Read the model definition and answer for the solid it produces. Units are mm, in the model's axes. A direction names the side the tool comes from. Give positions to 0.01 mm unless a question says otherwise; leave off trailing zeros. Write each loop counter-clockwise with the first axis right and the second up, starting at its lowest first coordinate (ties: lowest second). Pieces come first, ordered by that corner, then holes. Notation, with made-up numbers: (82, 61) -> (111, 61) arc R23 ccw to (111, 71) -> close; hole circle Ø11 at (14.25, 80.5). An arc over 180 degrees is marked (long way). Answer as CSV lines item,"result". Start each with the question number.
1. The part is cut by section B-B, the plane z = -36.5. Determine the outline of the cut face in (x, y), and give its area (3 significant figures).
2. Find the intervals of material crossed by line 1 (Z direction, x = 14.5, y = -16.5); line 2 (Y direction, x = -3.5, z = 11); line 3 (Y direction, x = -6.5, z = 0), in increasing order.
3. A tool of negligible diameter and unlimited length cuts with its end or side. For faces 1 (the flat face through (17, 0, 27)), 2 (the cylindrical face through (-19.535, 0.325, 29.423)), 3 (the cylindrical face through (0.325, 19.535, 29.423)), 4 (the flat face through (-7, -18, 32.845)), 5 (the cylindrical face through (-0.325, -19.535, 29.423)), from which of +Z, -Z, +X, -X, +Y, -Y can it reach the whole face along a straight path? Write none if from no direction.
4. Given pin 1 (6.5 mm diameter, centred on y = 0, z = 26.94, fed in from +X); pin 2 (2.5 mm diameter, centred on y = -1, z = 27, fed in from +X); pin 3 (4.5 mm diameter, centred on x = 0, z = 26.94, fed in from -Y); pin 4 (6 mm diameter, centred on x = -1, y = -1.5, fed in from +Z), each flat-ended and moving along its own axis, determine where each tip first touches the part or whether it passes through.
5. For a pull along X with two mould halves and no side action, classify faces 6 (the conical face through (10.92, -3.44, 23.22)), 7 (the cylindrical face through (19.535, -0.325, 29.423)), 8 (the cylindrical face through (20.32, 8.43, 26.24)) as pulls with the +X half, pulls with the -X half, needs draft (parallel to the pull), parting line crosses it, or undercut.
6. The part is cut by section A-A, the plane z = -15. Determine the outline of the cut face in (x, y).
from build123d import *

# Parameters (mm, degrees)
FILETE5_R             = 1
ESBO_O2_R             = 2.5
CORTE_EXTRUS_O1_DEPTH = 5
PADR_OCIRCULAR1_COUNT = 4
FILETE6_R             = 5
FILETE7_R             = 1
FILETE8_R             = 2


with BuildPart() as part:
    # Esbo_o1 → Revolu_o1 (revolve)
    with BuildSketch(Plane(origin=(0, 0, 0), x_dir=(1, 0, 0), z_dir=(0, 1, 0)), mode=Mode.PRIVATE) as revolu_o1_sk:
        Polygon((-7, -12.473975434), (-15, 48.292057468), (-18.025886882, 48.292057468), (-10.025886882, -12.473975434), (-22, -19.444538182), (-22, -32.844538182), (-19, -32.844538182), (-19, -36.444538182), (-22, -36.444538182), (-22, -41.444538182), (-19, -41.444538182), align=None)
    revolve(revolu_o1_sk.sketch.rotate(Axis((0, 0, 0), (0, 0, -1)), 180), axis=Axis((0, 0, 0), (0, 0, -1)))

    # Filete5
    filete5_edges = [part.edges().sort_by_distance(p)[0] for p in [
        (-7, 0, 12.473975434),
    ]]
    fillet(filete5_edges, radius=FILETE5_R)

    # Esbo_o2 → Corte-extrus_o1 (cut)
    with BuildSketch(Plane.ZX.offset(22)):
        with Locations(Location((26.944538182, 0, 0), (0, 0, 270))):
            Circle(ESBO_O2_R)
    corte_extrus_o1 = extrude(amount=-CORTE_EXTRUS_O1_DEPTH, mode=Mode.SUBTRACT)

    # Padr_oCircular1: Corte-extrus_o1 ×4 about axis
    padr_ocircular1_axis = Axis((0, 0, 0), (0, 0, 1))
    for i in range(1, PADR_OCIRCULAR1_COUNT):
        add(corte_extrus_o1.rotate(padr_ocircular1_axis, i * 360 / PADR_OCIRCULAR1_COUNT), mode=Mode.SUBTRACT)

    # Filete6
    filete6_edges = [part.edges().sort_by_distance(p)[0] for p in [
        (-10.025886882, 0, 12.473975434),
    ]]
    fillet(filete6_edges, radius=FILETE6_R)

    # Filete7
    filete7_edges = [part.edges().sort_by_distance(p)[0] for p in [
        (-18.025886882, 0, -48.292057468),
        (-15, 0, -48.292057468),
    ]]
    fillet(filete7_edges, radius=FILETE7_R)

    # Filete8
    filete8_edges = [part.edges().sort_by_distance(p)[0] for p in [
        (-19, 0, 41.444538182),
    ]]
    fillet(filete8_edges, radius=FILETE8_R)


solid = part.part
Results found:
1,outline,"circle Ø32.95 at (0, 0); hole circle Ø26.9 at (0, 0)"
1,area,"284 mm²"
2,line 1,"z = 19.42 to 32.84, 36.44 to 41.44"
2,line 2,"y = -9.96 to -6.29, 6.29 to 9.96"
2,line 3,"y = -9.69 to -5.7, 5.7 to 9.69"
3,face 1,"+X"
3,face 2,"-X"
3,face 3,"+Y"
3,face 4,"none"
3,face 5,"-Y"
4,pin 1,"stops at x = 22"
4,pin 2,"stops at x = 17"
4,pin 3,"stops at y = -17"
4,pin 4,"passes through"
5,face 6,"undercut"
5,face 7,"needs draft"
5,face 8,"parting line crosses it"
6,outline,"circle Ø27.29 at (0, 0); hole circle Ø21.23 at (0, 0)"
